The listing builds one solid part. Answer for the finished solid, in the listing's coordinates (mm). A direction names the side the tool comes from. Round coordinates to 2 decimals unless told otherwise and drop trailing zeros. Order: outer loops, then holes, each group sorted by start corner. A loop starts at its lowest first (then second) coordinate and runs counter-clockwise, first axis right, second up. Notation, with made-up numbers: (-25, -32) -> (-6, -32) arc R21 cw to (-6, -20) -> close; hole circle Ø10 at (39.25, -39). An arc over 180 degrees is marked (long way). Answer in a Markdown table with one row per item. Add a question column.
```python
from build123d import *

# Parameters (mm, degrees)
SKETCH1_R           = 2.805320717
SKETCH1_W           = 10.573901166
SKETCH1_H           = 9.926519461
BOSS_EXTRUDE1_DEPTH = 2.54


with BuildPart() as part:
    # Sketch1 → Boss-Extrude1 (new body)
    with BuildSketch(Plane(origin=(0, 0, 0), x_dir=(1, 0, 0), z_dir=(0, 1, 0))):
        with BuildLine():
            Line((70.780399637, 0), (-70.780399637, 0))
            ThreePointArc((-70.780399637, 0), (-76.832778265, 8.631756053), (-70.780399637, 17.263512107))
            Line((-70.780399637, 17.263512107), (-33.879642509, 23.089947443))
            Line((-33.879642509, 23.089947443), (-18.774069416, 35.390199818))
            Line((-18.774069416, 35.390199818), (18.774069416, 35.390199818))
            Line((18.774069416, 35.390199818), (33.879642509, 23.089947443))
            Line((33.879642509, 23.089947443), (70.780399637, 17.263512107))
            ThreePointArc((70.780399637, 17.263512107), (76.832778265, 8.631756053), (70.780399637, 0))
        make_face()
        with Locations(Location((-15.321366995, 29.455867532, 0), (0, 0, 270))):
            Circle(SKETCH1_R, mode=Mode.SUBTRACT)
        with Locations(Location((15.321366995, 29.455867532, 0), (0, 0, 90))):
            Circle(SKETCH1_R, mode=Mode.SUBTRACT)
        with Locations((0, 26.434752913)):
            Rectangle(SKETCH1_W, SKETCH1_H, mode=Mode.SUBTRACT)
    extrude(amount=BOSS_EXTRUDE1_DEPTH)


solid = part.part
```
1. The part is cut by section C-C (x = -39.5). Give the vertices of the cut face in (y, z), then the cut area to 3 significant figures.
2. The mould has two halves that part along Z. Classify faces 3 (the cylindrical face through (-76.83, 1.25, -8.47)), 4 (the flat face through (-52.588, 1.252, -20.136)), 5 (the flat face through (0, 1, -21.471)), 6 (the flat face through (1, 0, -14)): released by +Z, released by -Z, zero draft, split by the parting line, or undercut.
3. For faces 1 (the flat face through (-26.433, 1.252, -29.154)), 2 (the flat face through (-5.287, 1, -26)), determine the directions among +Z, -Z, +X, -X, +Y, -Y from which every point of the face is accessible in a straight line to the end or side of a thin tool.
4. Each of these flat-tipped pins is pushed along its axis until it touches: pin 1 (1.3 mm diameter, centred on y = 1, z = -24.5, fed in from +X); pin 2 (1 mm diameter, centred on x = -10, z = -25, fed in from -Y); pin 3 (5 mm diameter, centred on x = 15.32, z = -29.46, fed in from +Y); pin 4 (1 mm diameter, centred on x = 33.5, y = 2, fed in from -Z). Where does it stop, or does it pass through?
5. The part is cut by section A-A (y = 0.6). Give the vertices of the cut face in (x, z).
6. Straight lines are drawn through the part: line 1 along Z through (x, y) = (-15.5, 0.7); line 2 along X through (y, z) = (0.3, -31.5); line 3 along X through (y, z) = (0.35, -31). For each, find the intervals that lie inside material, in ascending order.
7. The part is cut by section B-B (x = 48.5). Give the vertices of the cut face in (y, z).
Report:
| question | item | result |
|---|---|---|
| 1 | outline | (0, -22.2) -> (2.54, -22.2) -> (2.54, 0) -> (0, 0) -> close |
| 1 | area | 56.4 mm^2 |
| 2 | face 3 | split by the parting line |
| 2 | face 4 | released by -Z |
| 2 | face 5 | undercut |
| 2 | face 6 | zero draft |
| 3 | face 1 | -Z, -X, +Y, -Y |
| 3 | face 2 | +Y, -Y |
| 4 | pin 1 | stops at x = 32.95 |
| 4 | pin 2 | stops at y = 0 |
| 4 | pin 3 | passes through |
| 4 | pin 4 | stops at z = -23.81 |
| 5 | outline | (-70.78, -17.26) -> (-33.88, -23.09) -> (-18.77, -35.39) -> (18.77, -35.39) -> (33.88, -23.09) -> (70.78, -17.26) arc R9.18 ccw to (70.78, 0) -> (-70.78, 0) arc R9.18 ccw to start; hole circle Ø5.61 at (-15.32, -29.46); hole (-5.29, -31.4) -> (5.29, -31.4) -> (5.29, -21.47) -> (-5.29, -21.47) -> close; hole circle Ø5.61 at (15.32, -29.46) |
| 6 | line 1 | z = -35.39 to -32.26, -26.66 to 0 |
| 6 | line 2 | x = -23.55 to -17.24, -13.4 to 13.4, 17.24 to 23.55 |
| 6 | line 3 | x = -24.17 to -17.66, -12.98 to -5.29, 5.29 to 12.98, 17.66 to 24.17 |
| 7 | outline | (0, -20.78) -> (2.54, -20.78) -> (2.54, 0) -> (0, 0) -> close |
